from build123d import *

# Parameters (mm, degrees)
F1_DEPTH = 254
F2_R     = 9.4654470454
F3_DEPTH = 64.1706123384
F4_T     = -2.54


# Not quite as in the source:
# - a shell that OpenCascade refuses in one call is made with other operations: the cavity is built on its own and cut out


with BuildPart() as f1:
    # F0 (on Front) → F1 (new body)
    with BuildSketch(Plane.XZ):
        with BuildLine():
            Line((-8.8068979187, 65.0390158129), (-27.5814907687, -0.52515852))
            ThreePointArc((-27.5814907687, -0.52515852), (0, -37.1132800896), (27.5814907687, -0.52515852))
            Line((27.5814907687, -0.52515852), (8.8068979187, 65.0390158129))
            ThreePointArc((8.8068979187, 65.0390158129), (0, 71.6779839596), (-8.8068979187, 65.0390158129))
        make_face()
    extrude(amount=F1_DEPTH)

    # F2 (on face) → F3 (cut, through all)
    with BuildSketch(Plane(origin=(25.3522532018, 0, 7.2597304326), x_dir=(0, 1, 0), z_dir=(0.961361214, 0, 0.2752900583))):
        with Locations((-127, 20.2662516385)):
            Circle(F2_R)
    extrude(amount=-F3_DEPTH, mode=Mode.SUBTRACT)

    # F4: a shell. OpenCascade refuses it in one call, so the cavity is built on its own and cut out:
    # the body offset inwards by the wall thickness, plus a prism from it out through each open face.
    f4_core = offset(f1.part, amount=F4_T, mode=Mode.PRIVATE)
    f4_exits = [f4_core.faces().sort_by_distance(p)[0] for p in [
        (24.429127, -127, 1.256817),
    ]]
    add(f4_core, mode=Mode.SUBTRACT)
    extrude(f4_exits, amount=-F4_T, mode=Mode.SUBTRACT)


solid = f1.part
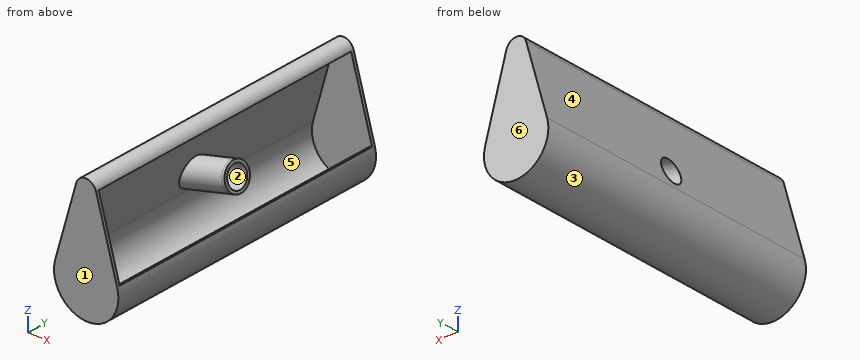
Build history of the part. All positions in model axes, mm. Face numbers are marked on the shaded views. A direction names the side the tool comes from. Round coordinates to 2 decimals unless told otherwise and drop trailing zeros. Write each loop counter-clockwise with the first axis right and the second up, starting at its lowest first coordinate (ties: lowest second). Pieces come first, ordered by that corner, then holes. Notation, with made-up numbers: M 36,-3.5 L 47,-3.5 A31 cw 47,35.5 Z; hole C 45,-10 d9. An arc over 180 degrees is marked long. Answer in a Markdown table with one row per item.
1. Saw through at A-A (y = -112). List the corners of the cut face in (x, z).
Geometry check:
| item | result |
|---|---|
| outline | M -27.58,-0.53 A28.69 ccw long 27.58,-0.53 L 25.14,-1.22 A26.15 cw long -25.14,-1.22 L -6.37,64.34 A6.62 cw 6.37,64.34 L 8.81,65.04 A9.16 ccw -8.81,65.04 Z |
2. Saw through at B-B (x = 0). State how many separate pieces and enclosed holes the cut face has, and give its area (3 significant figures).
Geometry check:
| item | result |
|---|---|
| separate pieces | 2 |
| enclosed holes | 2 |
| area | 2,000 mm2 |
3. Probe L1, parallel to Y at x = -11, z = 22.5; L2, parallel to X at y = -76.5, z = -9; L3, parallel to Y at x = 21.5, z = 10. List the from-to ranges inside material, lowest first. Write a range as [from, to].
Geometry check:
| item | result |
|---|---|
| L1 | [-254, -251.46], [-138.17, -135.38], [-118.62, -115.83], [-2.54, 0] |
| L2 | [-28.68, -26.14], [26.14, 28.68] |
| L3 | [-254, -251.46], [-2.54, 0] |
4. Flat gauge pins, fed straight in: P1, Ø8, axis at y = -138, z = 28.5, coming from the -X side; P2, Ø8, axis at y = -113.5, z = -17.5, coming from the +X side; P3, Ø8, axis at x = 15.5, y = -191.5, coming from the +Z side. Where does each tip first touch, or does it go through?
Geometry check:
| item | result |
|---|---|
| P1 | x = -20.42 |
| P2 | x = 28.24 |
| P3 | z = -25.85 |
5. Mould opens along X. For the marked faces 1, 2, 3 and 4 say: +X half, -X half, draft (parallel to the pull), parting line (faces both ways), or undercut.
Geometry check:
| item | result |
|---|---|
| face 1 | draft |
| face 2 | undercut |
| face 3 | parting line |
| face 4 | -X half |
6. Which spindle directions (+Z, -Z, +X, -X, +Y, -Y) get a long thin tool onto all of the face, cutting with end or side? Do the marked faces 5 and 6. Say none if no direction does.
Geometry check:
| item | result |
|---|---|
| face 5 | none |
| face 6 | +Z, -Z, +X, -X, +Y |
